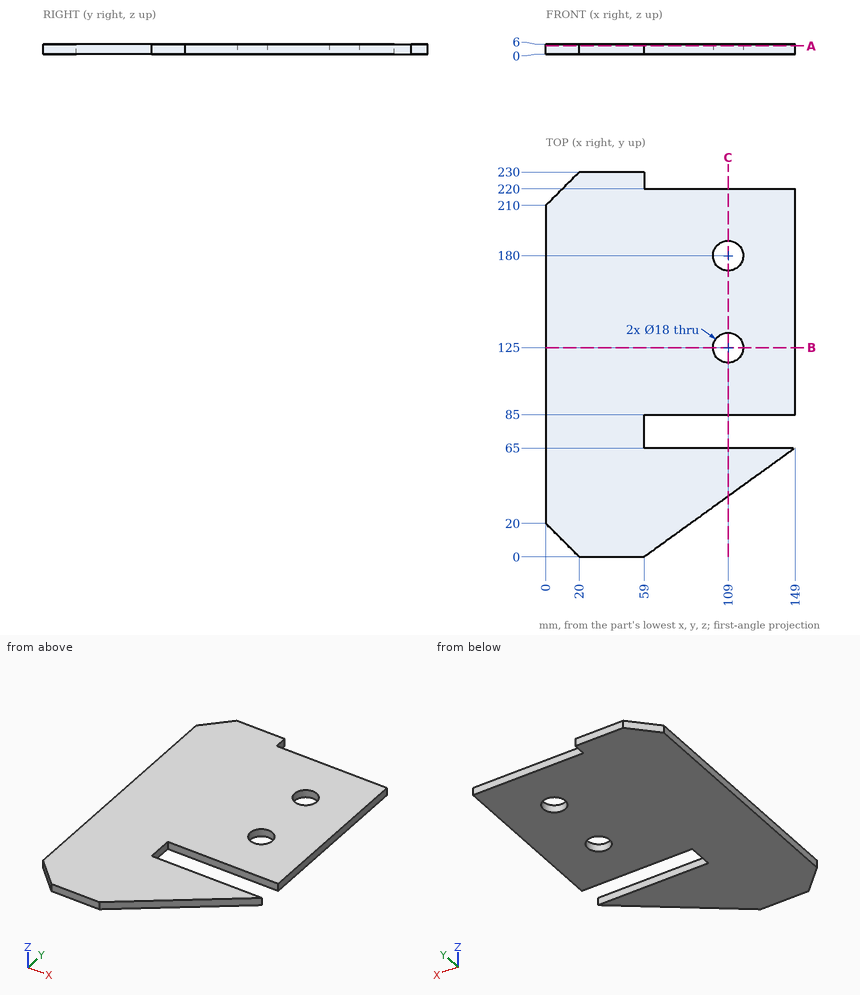
Verification items for this drawing (mm, ordinates from the low corner). Coordinates: 2 decimals unless noted, no trailing zeros. Write each loop counter-clockwise with the first axis right and the second up, starting at its lowest first coordinate (ties: lowest second). Pieces come first, ordered by that corner, then holes. Notation, with made-up numbers: M -40,17.5 L -13,17.5 A25 cw -13,35.5 Z; hole C 43,88.5 d8. An arc over 180 degrees is marked long. Answer as a JSON object with one key per item and string values.
1. Section check A-A, the plane z = 4.85. Enter the section's corners in (x, y).
Answers below:
{"outline": "M 0,20 L 20,0 L 59,0 L 149,65 L 59,65 L 59,85 L 149,85 L 149,220 L 59,220 L 59,230 L 20,230 L 0,210 Z; hole C 109,125 d18; hole C 109,180 d18"}
2. Scan lines: L1, parallel to Y at x = 114, z = 5; L2, parallel to Y at x = 109, z = 4.5; L3, parallel to X at y = 180, z = 2.65. Record each from-to range of solid material in increasing order.
Answers below:
{"L1": "y = 39.72 to 65, 85 to 117.52, 132.48 to 172.52, 187.48 to 220", "L2": "y = 36.11 to 65, 85 to 116, 134 to 171, 189 to 220", "L3": "x = 0 to 100, 118 to 149"}
3. Go/stop test with flat-tipped pins: pin 1 Ø2 at (x, z) = (91.5, 3.5) entering from +Y; pin 2 Ø1.8 at (x, z) = (91.5, 2) entering from -Y. Record where each tip stops, or that it passes through.
Answers below:
{"pin 1": "stops at y = 220", "pin 2": "stops at y = 22.82"}
4. Section check C-C, the plane x = 109. Enter the section's corners in (y, z), plus the area to 3 significant figures.
Answers below:
{"outline": "M 36.11,0 L 65,0 L 65,6 L 36.11,6 Z; M 85,0 L 116,0 L 116,6 L 85,6 Z; M 134,0 L 171,0 L 171,6 L 134,6 Z; M 189,0 L 220,0 L 220,6 L 189,6 Z", "area": "767 mm²"}
5. Section check B-B, the plane y = 125. Enter the section's corners in (x, z), plus the area to 3 significant figures.
Answers below:
{"outline": "M 0,0 L 100,0 L 100,6 L 0,6 Z; M 118,0 L 149,0 L 149,6 L 118,6 Z", "area": "786 mm²"}
